from build123d import *

# Parameters (mm, degrees)
F0_W      = 2438.4
F0_H      = 762
F1_DEPTH  = 3.4163
F2_W      = 2438.4
F2_H      = 762
F3_DEPTH  = 38.1
F4_W      = 38.1
F4_H      = 38.1
F5_DEPTH  = 800.1
F6_W      = 2438.4
F6_H      = 762
F6_W_2    = 1162.05
F6_H_2    = 685.8
F7_DEPTH  = 38.1
F10_DEPTH = 38.1


with BuildPart() as f1:
    # F0 (on Top) → F1 (new body)
    with BuildSketch(Plane.XY):
        Rectangle(F0_W, F0_H)
    extrude(amount=-F1_DEPTH)

    # F2 (on face) → F3 (join)
    with BuildSketch(Plane(origin=(0, 0, -3.4163), x_dir=(1, 0, 0), z_dir=(0, 0, -1))):
        Rectangle(F2_W, F2_H)
        Polygon((-600.075, -22.1201055787), (-56.5312900084, -342.9), (-1143.6187099916, -342.9), align=None, mode=Mode.SUBTRACT)
        Polygon((600.075, -22.1201055787), (1143.6187099916, -342.9), (56.5312900084, -342.9), align=None, mode=Mode.SUBTRACT)
        Polygon((19.05, -320.7798944213), (19.05, 320.7798944213), (562.5937099916, 0), align=None, mode=Mode.SUBTRACT)
        Polygon((-1181.1, -320.7798944213), (-1181.1, 320.7798944213), (-637.5562900084, 0), align=None, mode=Mode.SUBTRACT)
        Polygon((-562.5937099916, 0), (-19.05, 320.7798944213), (-19.05, -320.7798944213), align=None, mode=Mode.SUBTRACT)
        Polygon((-1143.6187099916, 342.9), (-56.5312900084, 342.9), (-600.075, 22.1201055787), align=None, mode=Mode.SUBTRACT)
        Polygon((56.5312900084, 342.9), (1143.6187099916, 342.9), (600.075, 22.1201055787), align=None, mode=Mode.SUBTRACT)
        Polygon((637.5562900084, 0), (1181.1, 320.7798944213), (1181.1, -320.7798944213), align=None, mode=Mode.SUBTRACT)
    extrude(amount=F3_DEPTH)

    # F4 (on face) → F5 (join)
    with BuildSketch(Plane(origin=(0, 0, -41.5163), x_dir=(1, 0, 0), z_dir=(0, 0, -1))):
        with Locations((-1200.15, 361.95)):
            Rectangle(F4_W, F4_H)
        with Locations((-1200.15, -361.95)):
            Rectangle(F4_W, F4_H)
        with Locations((1200.15, -361.95)):
            Rectangle(F4_W, F4_H)
        with Locations((1200.15, 361.95)):
            Rectangle(F4_W, F4_H)
    extrude(amount=F5_DEPTH)

    # F6 (on face) → F7 (join)
    with BuildSketch(Plane(origin=(0, 0, -841.6163), x_dir=(1, 0, 0), z_dir=(0, 0, -1))):
        Rectangle(F6_W, F6_H)
        with Locations((-600.075, 0)):
            Rectangle(F6_W_2, F6_H_2, mode=Mode.SUBTRACT)
        with Locations((600.075, 0)):
            Rectangle(F6_W_2, F6_H_2, mode=Mode.SUBTRACT)
    extrude(amount=F7_DEPTH)

    # F9 (on 3pt) → F10 (join)
    with BuildSketch(Plane(origin=(0, 381, 0), x_dir=(-1, 0, 0), z_dir=(0, 1, 0))):
        Polygon((19.05, -818.4874808139), (19.05, -41.5163), (-19.05, -41.5163), (-19.05, -818.4874808139), (-1147.508143563, -41.5163), (-1181.1, -41.5163), (-1181.1, -64.645119186), (-52.6418564368, -841.6163), (-19.05, -841.6163), (19.05, -841.6163), (52.6418564369, -841.6163), (1181.1, -64.6451191861), (1181.1, -41.5163), (1147.5081435631, -41.5163), align=None)
    extrude(amount=-F10_DEPTH)


solid = f1.part
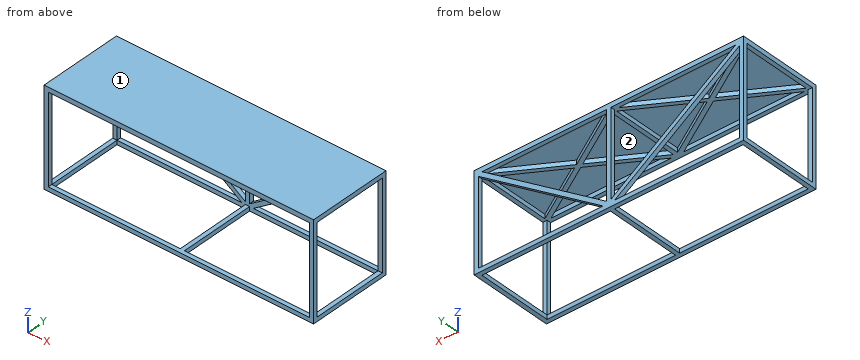
The listing builds one solid part. Answer for the finished solid, in the listing's coordinates (mm). Face numbers are marked on the shaded views. Coordinates: 2 decimals unless noted, no trailing zeros. Loops run counter-clockwise (first coordinate to the right, second up) from the corner with the lowest first, then second, coordinate; pieces in that order, holes last.
1) Find section A-A on x = 862.5. Write down the section's boundary in (y, z), then the cut area to 3 significant figures.
2) Determine the mould class of the marked faces 1 and 2 for opening direction X: pulls with the +X half, pulls with the -X half, needs draft (parallel to the pull), parting line crosses it, or undercut.
3) A flat-ended cylindrical pin translates along its axis: pin 1 Ø10 at (x, y) = (316.5, -111) entering from +Z. Find the tip coordinate at first contact, or state that the pin passes through.
4) Find the intervals of material crossed by L1, parallel to Z at x = 412, y = -348.5; L2, parallel to Y at x = 457.5, z = -540; L3, parallel to Z at x = -458.5, y = 133, in increasing order.
5) Find section C-C on y = 177.5. Give the number of separate pieces and of enclosed holes in the cut face, then the cut area to 3 significant figures.
6) Find section B-B on z = -548.5. Write down the section's boundary in (x, y), then the cut area to 3 significant figures.
Values:
1. outline: (-381, -879.72) - (-342.9, -879.72) - (-342.9, -841.62) - (-381, -841.62) - close; (-381, -41.52) - (-342.9, -41.52) - (-342.9, -3.42) - (-176.99, -3.42) - (-176.99, -41.52) - (-132.75, -41.52) - (-132.75, -3.42) - (132.75, -3.42) - (132.75, -41.52) - (176.99, -41.52) - (176.99, -3.42) - (342.9, -3.42) - (342.9, -41.52) - (381, -41.52) - (381, 0) - (-381, 0) - close; (342.9, -879.72) - (381, -879.72) - (381, -841.62) - (342.9, -841.62) - close; (342.9, -284.01) - (381, -284.01) - (381, -237.75) - (342.9, -237.75) - close
1. area: 13,500 mm2
2. face 1: needs draft
2. face 2: undercut
3. pin 1: stops at z = 0
4. L1: z = -879.72 to -841.62, -41.52 to 0
4. L2: y = 342.9 to 381
4. L3: z = -3.42 to 0
5. separate pieces: 4
5. enclosed holes: 0
5. area: 28,500 mm2
6. outline: (-1219.2, -381) - (-1181.1, -381) - (-1181.1, -342.9) - (-1219.2, -342.9) - close; (-1219.2, 342.9) - (-1181.1, 342.9) - (-1181.1, 381) - (-1219.2, 381) - close; (-478.36, 342.9) - (-411.17, 342.9) - (-411.17, 381) - (-478.36, 381) - close; (-19.05, 342.9) - (19.05, 342.9) - (19.05, 381) - (-19.05, 381) - close; (411.17, 342.9) - (478.36, 342.9) - (478.36, 381) - (411.17, 381) - close; (1181.1, -381) - (1219.2, -381) - (1219.2, -342.9) - (1181.1, -342.9) - close; (1181.1, 342.9) - (1219.2, 342.9) - (1219.2, 381) - (1181.1, 381) - close
6. area: 12,400 mm2
